Design review of the part built by this model. Coordinates are the model's own, in mm. Give positions to 0.01 mm unless a question says otherwise; leave off trailing zeros. Write each loop counter-clockwise with the first axis right and the second up, starting at its lowest first coordinate (ties: lowest second). Pieces come first, ordered by that corner, then holes. Notation, with made-up numbers: M 41.5,11.25 L 45.5,11.25 A24 ccw 45.5,45.25 Z; hole C -20,-31 d3. An arc over 180 degrees is marked long. One line per item, written item: value. Start each with the question number.
Autodesk Inventor part; units mm, degrees
ref_plane "YZ Plane" through (0, 0, 0) normal (1, 0, 0) x (0, 1, 0)
ref_plane "XZ Plane" through (0, 0, 0) normal (0, 1, 0) x (-1, 0, 0)
ref_plane "XY Plane" through (0, 0, 0) normal (0, 0, 1) x (1, 0, 0)
sketch "Sketch1" plane through (0, 0, 0) normal (0, 1, 0) x (-1, 0, 0)
  line L0 (0, 0) -> (200, 0)
  line L1 (200, 0) -> (200, -60)
  line L2 (200, -60) -> (0, -60)
  line L3 (0, -60) -> (0, 0)
  dimension "d0" = 200
  dimension "d1" = 60
extrude "Extrusion1" add sketch "Sketch1" along normal blind 8
sketch "Sketch2" plane through (0, 8, 0) normal (0, 1, 0) x (1, 0, 0)
  line L0 (-40, 7.5) -> (-40, 52.5)
  line L1 (-35, 42.75) -> (-35, 34.25)
  line L2 (-35, 34.25) -> (-34, 34.25)
  line L3 (-34, 34.25) -> (-34, 42.75)
  line L4 (-34, 42.75) -> (-35, 42.75)
  line L5 (-34, 25.75) -> (-35, 25.75)
  line L6 (-35, 25.75) -> (-35, 17.25)
  line L7 (-35, 17.25) -> (-34, 17.25)
  line L8 (-34, 17.25) -> (-34, 25.75)
  line L9 (-40, 7.5) -> (-5, 7.5)
  line L10 (-5, 52.5) -> (-40, 52.5)
  line L11 (-23.5275, 30) -> (-17.7049, 30) construction
  line L12 (-5, 52.5) -> (-5, 7.5)
  circle A0 centre (-36, 11.5) radius 1.5
  circle A1 centre (-9, 11.5) radius 1.5
  circle A2 centre (-36, 48.5) radius 1.5
  circle A3 centre (-9, 48.5) radius 1.5
  line L13 (-200, 0) -> (0, 0) construction
  line L14 (0, 0) -> (0, 60) construction
  point P0 (-35.5, 13)
  point P1 (-35.5, 30)
  point P2 (-35.5, 47)
  dimension "d4" = 8.5
  dimension "d5" = 1
  dimension "d6" = 5
  dimension "d7" = 17
  dimension "d8" = 17
  dimension "d9" = 4.25
  dimension "d10" = 4.25
  dimension "d11" = 4.5
  dimension "d12" = 35
  dimension "d13" = 45
  dimension "d14" = 3
  dimension "d15" = 4
  dimension "d16" = 4
  dimension "d17" = 4
  dimension "d18" = 4
  dimension "d19" = 7.5
  dimension "d20" = 5
hole "Hole1" at (-36, 8, -11.5) at (-36, 8, -48.5) at (-9, 8, -11.5) at (-9, 8, -48.5) direction (0, -1, 0) diameter 4 end through all
properties part number "Base"
Q1. Take a section at B-B, the plane x = -9. Give the boundary of the cut face in (y, z).
Q2. Wall thickness on line 1 (X direction, y = 3.5, z = -11.5); line 2 (Z direction, x = -9, y = 4); line 3 (X direction, y = 6.75, z = -13): over which ranges is each line inside the solid? List them lowest first. Write a range as from..to.
Q3. Take a section at A-A, the plane z = -48.5. Give the boundary of the cut face in (x, y), then the cut area to 3 significant figures.
Q4. The part is to be moulded in two halves that separate along Z. For faces 1 (the face through (-34.048, 3.944, -48.934)), 2 (the face through (-101, 4, -60)), 3 (the face through (-99, 8, -30)), say which applies: pulls with the +Z half, pulls with the -Z half, needs draft (parallel to the pull), parting line crosses it, or undercut.
Results list:
1. outline: M 0,-60 L 8,-60 L 8,-50.5 L 0,-50.5 Z; M 0,-46.5 L 8,-46.5 L 8,-13.5 L 0,-13.5 Z; M 0,-9.5 L 8,-9.5 L 8,0 L 0,0 Z
2. line 1: x = -200..-38, -34..-11, -7..0
2. line 2: z = -60..-50.5, -46.5..-13.5, -9.5..0
2. line 3: x = -200..-37.32, -34.68..-10.32, -7.68..0
3. outline: M -200,0 L -38,0 L -38,8 L -200,8 Z; M -34,0 L -11,0 L -11,8 L -34,8 Z; M -7,0 L 0,0 L 0,8 L -7,8 Z
3. area: 1,540 mm^2
4. face 1: undercut
4. face 2: pulls with the -Z half
4. face 3: needs draft
